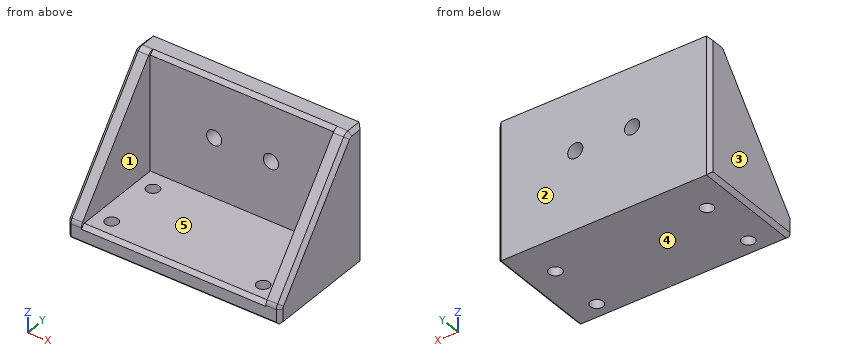
from build123d import *

# Parameters (mm, degrees)
SKETCH_1_W          = 39
SKETCH_1_H          = 29
SKETCH_1_R          = 1.6
EXTRUDE_1_DEPTH     = 4
SKETCH_2_W          = 39
SKETCH_2_H          = 4
EXTRUDE_2_DEPTH     = 20
SKETCH_3_R          = 1.35
CUT_EXTRUDE_1_DEPTH = 4
EXTRUDE_3_DEPTH     = 3
CHAMFER_1_SIZE      = 0.8
FILLET_1_R          = 1.6
CHAMFER_3_SIZE      = 0.8


with BuildPart() as part:
    # 草图1 → 凸台-拉伸1 (new body)
    with BuildSketch(Plane(origin=(0, 0, 0), x_dir=(1, 0, 0), z_dir=(0, 1, 0))):
        Rectangle(SKETCH_1_W, SKETCH_1_H)
        with Locations(Location((-6, -2, 0), (0, 0, 270))):
            Circle(SKETCH_1_R, mode=Mode.SUBTRACT)
        with Locations(Location((6, -2, 0), (0, 0, 90))):
            Circle(SKETCH_1_R, mode=Mode.SUBTRACT)
    extrude(amount=EXTRUDE_1_DEPTH)

    # 草图2 → 凸台-拉伸2 (add)
    with BuildSketch(Plane(origin=(0, 0, 0), x_dir=(-1, 0, 0), z_dir=(0, -1, 0))):
        with Locations((0, 12.5)):
            Rectangle(SKETCH_2_W, SKETCH_2_H)
    extrude(amount=EXTRUDE_2_DEPTH)

    # 草图3 → 切除-拉伸1 (cut)
    with BuildSketch(Plane.XY.offset(-10.5)):
        with Locations((16, -4)):
            Circle(SKETCH_3_R)
        with Locations(Location((16, -16, 0), (0, 0, 180))):
            Circle(SKETCH_3_R)
        with Locations((-16, -16)):
            Circle(SKETCH_3_R)
        with Locations(Location((-16, -4, 0), (0, 0, 180))):
            Circle(SKETCH_3_R)
    extrude(amount=-CUT_EXTRUDE_1_DEPTH, mode=Mode.SUBTRACT)

    # 草图4 → 凸台-拉伸3 (add)
    with BuildSketch(Plane(origin=(19.5, 0, 0), x_dir=(0, 0, -1), z_dir=(1, 0, 0))):
        Polygon((-14.5, 0), (10.5, -20), (14.5, -20), (14.5, 4), (-14.5, 4), align=None)
    extrude_3 = extrude(amount=EXTRUDE_3_DEPTH)

    # 镜向1: 凸台-拉伸3 across plane
    add(extrude_3.mirror(Plane(origin=(0, 0, 0), x_dir=(0, 0, 1), z_dir=(1, 0, 0))))

    # 倒角1
    chamfer_1_edges = [part.edges().sort_by_distance(p)[0] for p in [
        (0, -20, -10.5),
        (0, -20, -14.5),
        (0, 0, 14.5),
        (22.5, -8, -14.5),
        (22.5, 4, 0),
        (-22.5, 4, 0),
        (-22.5, -8, -14.5),
    ]]
    chamfer(chamfer_1_edges, length=CHAMFER_1_SIZE)

    # 圆角1
    fillet_1_edges = [part.edges().sort_by_distance(p)[0] for p in [
        (21, 0, 14.5),
        (21, -20, -10.5),
        (-21, 0, 14.5),
        (-21, -20, -10.5),
    ]]
    fillet(fillet_1_edges, radius=FILLET_1_R)

    # 倒角3
    chamfer_3_edges = [part.edges().sort_by_distance(p)[0] for p in [
        (22.5, 1.984499878, 14.5),
        (22.5, -20, -12.380624847),
        (22.5, 0.075897787, 14.342085178),
        (22.5, -19.909805311, -10.531638589),
        (22.5, -10.064890217, 1.918887229),
        (-22.5, -20, -12.380624847),
        (-22.5, -19.909805311, -10.531638589),
        (-22.5, -10.064890217, 1.918887229),
        (-22.5, 0.075897787, 14.342085178),
        (-22.5, 1.984499878, 14.5),
    ]]
    chamfer(chamfer_3_edges, length=CHAMFER_3_SIZE)


solid = part.part
Work out the finished part from the listing and answer in its coordinate system (mm). Face numbers are marked on the shaded views. A direction names the side the tool comes from. Coordinates: 2 decimals unless noted, no trailing zeros. Write each loop counter-clockwise with the first axis right and the second up, starting at its lowest first coordinate (ties: lowest second). Pieces come first, ordered by that corner, then holes. Notation, with made-up numbers: (-9.75, 85.25) - (-1.75, 85.25) arc R23 cw to (-1.75, 108.25) - close; hole circle Ø1 at (14.5, 2). An arc over 180 degrees is marked (long way). One line per question, with ' | ' between items.
1) Flat-ended cylindrical pins translate along their axes: P1, Ø3.5, axis at x = -16, y = -4, coming from the +Z side; P2, Ø6, axis at x = -7, z = -4.5, coming from the -Y side; P3, Ø10.5, axis at y = -12.5, z = 2.5, coming from the -X side. Find the tip coordinate at first contact, or state that the pin passes through.
Checks:
P1: z = -10.5 | P2: y = 0 | P3: x = -22.5
2) For the marked faces 4 and 5, determine the directions among +Z, -Z, +X, -X, +Y, -Y from which every point of the face is accessible in a straight line to the end or side of a thin tool.
Checks:
face 4: -Z, +X, -X, +Y, -Y | face 5: +Z, -Y
3) Find section D-D, the plane z = 2. Determine the outline of the cut face in (x, y), and give its area (3 significant figures).
Checks:
outline: (-22.5, -8.98) - (-21.7, -10) - (-19.5, -10) - (-19.5, 0) - (-7.6, 0) - (-7.6, 4) - (-21.7, 4) - (-22.5, 3.2) - close; (-4.4, 0) - (4.4, 0) - (4.4, 4) - (-4.4, 4) - close; (7.6, 0) - (19.5, 0) - (19.5, -10) - (21.7, -10) - (22.5, -8.98) - (22.5, 3.2) - (21.7, 4) - (7.6, 4) - close | area: 213 mm2
4) The mould has two halves that part along X. Classify the marked faces 1, 2 and 3: +X half, -X half, draft (parallel to the pull), parting line (faces both ways), or undercut.
Checks:
face 1: undercut | face 2: draft | face 3: -X half
5) Find section C-C, the plane x = -6. Determine the outline of the cut face in (y, z).
Checks:
outline: (-20, -13.7) - (-19.2, -14.5) - (4, -14.5) - (4, 0.4) - (0, 0.4) - (0, -10.5) - (-19.2, -10.5) - (-20, -11.3) - close; (0, 3.6) - (4, 3.6) - (4, 14.5) - (0.8, 14.5) - (0, 13.7) - close
6) Find section B-B, the plane y = -16. Determine the outline of the cut face in (x, z).
Checks:
outline: (-22.5, -13.7) - (-21.7, -14.5) - (-17.35, -14.5) - (-17.35, -10.5) - (-19.5, -10.5) - (-19.5, -5.5) - (-21.7, -5.5) - (-22.5, -6.78) - close; (-14.65, -14.5) - (14.65, -14.5) - (14.65, -10.5) - (-14.65, -10.5) - close; (17.35, -14.5) - (21.7, -14.5) - (22.5, -13.7) - (22.5, -6.78) - (21.7, -5.5) - (19.5, -5.5) - (19.5, -10.5) - (17.35, -10.5) - close
7) Consider probe 1 along Y at (x, z) = (16, -11.8); probe 2 along X at (y, z) = (-8.5, -2.5); probe 3 along Z at (x, y) = (6, 1.6). Determine where each line is inside the solid, lowest interval first. Write a range as [from, to].
Checks:
probe 1: [-20, -17.35], [-14.65, -5.35], [-2.65, 4] | probe 2: [-22.5, -19.5], [19.5, 22.5] | probe 3: [-14.5, 0.4], [3.6, 14.5]
8) Find section A-A, the plane x = -16. Determine the outline of the cut face in (y, z), and give its area (3 significant figures).
Checks:
outline: (-20, -13.7) - (-19.2, -14.5) - (-17.35, -14.5) - (-17.35, -10.5) - (-19.2, -10.5) - (-20, -11.3) - close; (-14.65, -14.5) - (-5.35, -14.5) - (-5.35, -10.5) - (-14.65, -10.5) - close; (-2.65, -14.5) - (4, -14.5) - (4, 14.5) - (0.8, 14.5) - (0, 13.7) - (0, -10.5) - (-2.65, -10.5) - close | area: 173 mm2
